Autodesk Fusion 360 part; units mm, degrees
sketch "Sketch1" plane through (0, 0, 0) normal (0, 1, 0) x (1, 0, 0)
  circle A0 centre (0, 0) radius 3
  dimension "d1" = 6
extrude "Extrude1" add sketch "Sketch1" along normal blind 10
sketch "Sketch2" plane through (0, 10, 0) normal (0, 1, 0) x (-1, 0, 0)
  circle A0 centre (0, 0) radius 3
  line L0 (0, 0) -> (-3, 0) construction
  line L1 (-3, 0) -> (-0.5, 0)
  line L2 (-0.5, 0) -> (1.5, 0)
  line L3 (1.5, 0) -> (3, 0)
  line L4 (1.5, 3) -> (-0.5, 3)
  line L5 (-0.5, 3) -> (-0.5, -3)
  line L6 (-0.5, -3) -> (1.5, -3)
  line L7 (1.5, -3) -> (1.5, 3)
  line L8 (1.5, 3) -> (-0.5, -3) construction
  line L9 (-0.5, 3) -> (1.5, -3) construction
  point P0 (0.5, 0)
  dimension "d4" = 2.5
  dimension "d5" = 2
  dimension "d6" = 2
  dimension "d7" = 6
extrude "Extrude2" add sketch "Sketch2" along normal blind 3 contours A0 L2 L5 L7 | A0 L4 L7 | A0 L6 L7 | A0 L2 L5 L7
extrude "Extrude3" add 2 faces at (-1.3827, 10, 2.7899) (-1.3827, 10, -2.7899) along direction (0, -1, 0) blind 3
fillet "Fillet1" radius 0.5 1 edges at (-2.797, 0, 1.0848)
Here's how the part is built. I have some questions about the finished solid (model axes, mm). A direction names the side the tool comes from. Round coordinates to 2 decimals unless told otherwise and drop trailing zeros. Order: outer loops, then holes, each group sorted by start corner. A loop starts at its lowest first (then second) coordinate and runs counter-clockwise, first axis right, second up. Notation, with made-up numbers: M -38,25 L -6,25 A29 ccw -6,49 Z; hole C -18.5,-10.75 d10. An arc over 180 degrees is marked long. Return JSON: item names as keys, results as strings. Group by question number.
1. On a 3-axis mill with a long thin cutter (end or side, diameter ignored), from which of +Z, -Z, +X, -X, +Y, -Y can I reach the whole of each face in a straight line? I mean faces 1 (the face through (-2, 10, 0)), 2 (the face through (-1, 10, -3)), 3 (the face through (0.5, 11, 0)), 4 (the face through (2.77, 5.27, -1.15)), 5 (the face through (0, 13, 0)). Say none if no direction works.
2. Please list where these lines run through material, in increasing order: probe 1 along X at (y, z) = (11.75, -0.3); probe 2 along Z at (x, y) = (0.1, 6); probe 3 along Y at (x, z) = (1.45, 1.35).
3. If we section it at A-A on z = 0: List the corners of the cut face in (x, y) for me.
4. I'm going to push flat-ended pins straight in: pin 1 Ø1.6 at (x, z) = (-2.5, -1) entering from +Y; pin 2 Ø3.5 at (y, z) = (12, 0) entering from +X; pin 3 Ø1 at (x, y) = (1.5, 5.5) entering from +Z. Where does each tip first touch, or does it pass through?
5. If we section it at B-B on y = 8.5: List the corners of the cut face in (x, z) for me.
Reply:
{
 "1": {"face 1": "+Z, -Z, -X, +Y", "face 2": "-Z, +X, -X, +Y, -Y", "face 3": "+Z, -Z, +X, +Y", "face 4": "-Y", "face 5": "+Z, -Z, +X, -X, +Y"},
 "2": {"probe 1": "-1.5 to 0.5", "probe 2": "-3 to 3", "probe 3": "0 to 10"},
 "3": {"outline": "M -3,0.5 A0.5 ccw -2.5,0 L 2.5,0 A0.5 ccw 3,0.5 L 3,10 L 0.5,10 L 0.5,13 L -1.5,13 L -1.5,10 L -3,10 Z"},
 "4": {"pin 1": "y = 10", "pin 2": "x = 0.5", "pin 3": "z = 2.83"},
 "5": {"outline": "M -1.5,-3 L 0,-3 A3 ccw 0,3 L -1.5,3 L -1.5,2.6 A3 ccw -1.5,-2.6 Z"}
}
